```python
from build123d import *

# Parameters (mm, degrees)
F0_R     = 56
F1_DEPTH = 10
F2_R     = 11.5
F3_DEPTH = 6
F5_DEPTH = 16
F6_R     = 2.2
F7_DEPTH = 10
F9_DEPTH = 5


with BuildPart() as f1:
    # F0 (on Top) → F1 (new body)
    with BuildSketch(Plane.XY):
        Circle(F0_R)
    extrude(amount=F1_DEPTH)

    # F2 (on face) → F3 (join)
    with BuildSketch(Plane.XY.offset(10)):
        Circle(F2_R)
    extrude(amount=F3_DEPTH)

    # F4 (on face) → F5 (cut)
    with BuildSketch(Plane.XY.offset(16)):
        with BuildLine():
            Line((2.833725, 3.1), (-2.833725, 3.1))
            ThreePointArc((-2.833725, 3.1), (0, -4.2), (2.833725, 3.1))
        make_face()
    extrude(amount=-F5_DEPTH, mode=Mode.SUBTRACT)

    # F6 (on face) → F7 (cut)
    with BuildSketch(Plane.XY.offset(10)):
        with Locations((0, 35)):
            Circle(F6_R)
        with Locations((35, 0)):
            Circle(F6_R)
        with Locations((-35, 0)):
            Circle(F6_R)
        with Locations((0, -35)):
            Circle(F6_R)
    extrude(amount=-F7_DEPTH, mode=Mode.SUBTRACT)

    # F8 (on face) → F9 (cut)
    with BuildSketch(Plane.XY.offset(10)):
        Polygon((3.6, 32.921539), (3.6, 37.078461), (0, 39.156922), (-3.6, 37.078461), (-3.6, 32.921539), (0, 30.843078), align=None)
        Polygon((38.6, -2.078461), (38.6, 2.078461), (35, 4.156922), (31.4, 2.078461), (31.4, -2.078461), (35, -4.156922), align=None)
        Polygon((3.6, -37.078461), (3.6, -32.921539), (0, -30.843078), (-3.6, -32.921539), (-3.6, -37.078461), (0, -39.156922), align=None)
        Polygon((-31.4, -2.078461), (-31.4, 2.078461), (-35, 4.156922), (-38.6, 2.078461), (-38.6, -2.078461), (-35, -4.156922), align=None)
    extrude(amount=-F9_DEPTH, mode=Mode.SUBTRACT)


solid = f1.part
```
Check sheet for the modelled part. Datum: model origin and axes. Units: mm. A direction names the side the tool comes from. Give positions to 0.01 mm unless a question says otherwise; leave off trailing zeros. Order: outer loops, then holes, each group sorted by start corner. A loop starts at its lowest first (then second) coordinate and runs counter-clockwise, first axis right, second up. Notation, with made-up numbers: M 32,12.25 L 68,12.25 A15 ccw 68,35.25 Z; hole C -39,37.5 d9. An arc over 180 degrees is marked long. Answer in a Markdown table with one row per item. Add a question column.
Q1. Sectioned sample at C-C, the plane x = -13.5. Record the boundary of the cut face in (y, z), and give its area (3 significant figures).
Q2. Gauge pin test, flat ends, axial feed: pin 1 Ø6 at (x, z) = (-1.5, 6.5) entering from -Y; pin 2 Ø6 at (y, z) = (-14, 4) entering from +X; pin 3 Ø2 at (y, z) = (-13, 2.5) entering from +X. Record the tip position at first contact, or that the pin passes through.
Q3. Access from +Z, -Z, +X, -X, +Y, -Y to the whole of each face (thin tool, end or side, straight path). Record for faces 1 (the cylindrical face through (-37.198, 0.097, 2.535)), 2 (the flat face through (-37, -2, 5)).
Q4. Thickness scan on L1, parallel to Y at x = 0, z = 5.5; L2, parallel to Y at x = 0, z = 1.2; L3, parallel to Z at x = -26, y = -47.5. Record the ranges inside material, lowest first.
Q5. Sectioned sample at A-A, the plane y = 0. Record the boundary of the cut face in (x, z).
Q6. Sectioned sample at D-D, the plane y = -13. Record the boundary of the cut face in (x, z).
Q7. Release check for a two-part mould opening along X. For faces 3 (the cylindrical face through (32.802, 0.097, 2.535)), 4 (the flat face through (12, 1, 10)) record: released by +X, released by -X, zero draft, split by the parting line, or undercut.
Q8. Sectioned sample at B-B, the plane y = -35. Record the boundary of the cut face in (x, z), and give its area (3 significant figures).
Verdict:
| question | item | result |
|---|---|---|
| 1 | outline | M -54.35,0 L 54.35,0 L 54.35,10 L -54.35,10 Z |
| 1 | area | 1,090 mm² |
| 2 | pin 1 | y = -56 |
| 2 | pin 2 | x = 54.91 |
| 2 | pin 3 | x = 54.7 |
| 3 | face 1 | +Z, -Z |
| 3 | face 2 | +Z |
| 4 | L1 | -56 to -39.16, -30.84 to -4.2, 3.1 to 30.84, 39.16 to 56 |
| 4 | L2 | -56 to -37.2, -32.8 to -4.2, 3.1 to 32.8, 37.2 to 56 |
| 4 | L3 | 0 to 10 |
| 5 | outline | M -56,0 L -37.2,0 L -37.2,5 L -38.6,5 L -38.6,10 L -56,10 Z; M -32.8,0 L -4.2,0 L -4.2,16 L -11.5,16 L -11.5,10 L -31.4,10 L -31.4,5 L -32.8,5 Z; M 4.2,0 L 32.8,0 L 32.8,5 L 31.4,5 L 31.4,10 L 11.5,10 L 11.5,16 L 4.2,16 Z; M 37.2,0 L 56,0 L 56,10 L 38.6,10 L 38.6,5 L 37.2,5 Z |
| 6 | outline | M -54.47,0 L 54.47,0 L 54.47,10 L -54.47,10 Z |
| 7 | face 3 | undercut |
| 7 | face 4 | zero draft |
| 8 | outline | M -43.71,0 L -2.2,0 L -2.2,5 L -3.6,5 L -3.6,10 L -43.71,10 Z; M 2.2,0 L 43.71,0 L 43.71,10 L 3.6,10 L 3.6,5 L 2.2,5 Z |
| 8 | area | 816 mm² |
